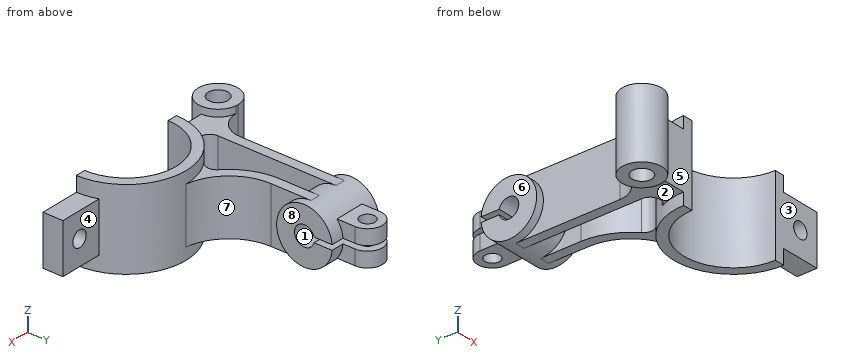
```python
from build123d import *

# Parameters (mm, degrees)
BOSS_EXTRUDE1_DEPTH = 40
SKETCH1_3_R         = 9.999999999999993
BOSS_EXTRUDE2_DEPTH = 35
BOSS_EXTRUDE3_DEPTH = 28
BOSS_EXTRUDE4_DEPTH = 25
SKETCH3_R           = 8.000000000000012
CUT_EXTRUDE1_DEPTH  = 67
SKETCH8_R           = 27.999999999999996
BOSS_EXTRUDE5_DEPTH = 28
SKETCH9_R           = 7.500000000000014
BOSS_EXTRUDE6_DEPTH = 17.5
SKETCH10_R          = 10.000000000000004
CUT_EXTRUDE3_DEPTH  = 60
SKETCH10_4_R        = 10.000000000000004
CUT_EXTRUDE4_DEPTH  = 60


with BuildPart() as part:
    # Sketch1 → Boss-Extrude1 (new, symmetric)
    with BuildSketch(Plane.XY):
        with BuildLine():
            ThreePointArc((50, 0), (3.06e-15, 50), (-50, 0))
            Line((-50, 0), (-60, 0))
            ThreePointArc((-60, 0), (3.67e-15, 60), (60, 0))
            Line((60, 0), (50, 0))
        make_face()
    extrude(amount=BOSS_EXTRUDE1_DEPTH, both=True)



with BuildPart() as body_2:
    # Sketch1<3> → Boss-Extrude2 (new, symmetric)
    with BuildSketch(Plane.XY):
        with BuildLine():
            ThreePointArc((-110, 19.999999999999986), (-124.14213562373095, -14.142135623730939), (-90.00000000000001, -4.9e-15))
            ThreePointArc((-90.00000000000001, 0), (-95.13196534092553, 13.376903430037897), (-107.894154537656, 19.88882638288958))
            ThreePointArc((-107.894154537656, 19.888826382889572), (-108.94824999295787, 19.92219950575522), (-110, 20))
        make_face()
        with Locations((-110, 0)):
            Circle(SKETCH1_3_R, mode=Mode.SUBTRACT)
    extrude(amount=BOSS_EXTRUDE2_DEPTH, both=True)


with BuildPart() as part_1:
    add(part.part)

    add(body_2.part)  # Boss-Extrude3 merges body 2
    # Sketch1<6> → Boss-Extrude3 (add, symmetric)
    with BuildSketch(Plane.XY):
        with BuildLine():
            ThreePointArc((-32.98168393227754, 65.04935068656462), (-29.729511757993123, 56.976796834196755), (-34.03450339822838, 49.413081045771484))
            ThreePointArc((-34.034503398228374, 49.413081045771484), (-17.821547874044366, 57.29216727767544), (-1.66e-15, 59.99999999999999))
            ThreePointArc((-1.78e-15, 59.99999999999999), (-30.50166992482464, 76.80795981518852), (-42.63026373834409, 109.45388748555197))
            Line((-42.630263738344084, 109.45388748555196), (-42.63026373834409, 150))
            Line((-42.63026373834409, 150), (-52.63026373834409, 150))
            Line((-52.63026373834409, 150), (-52.63026373834409, 139.99999999999997))
            Line((-52.63026373834409, 139.99999999999997), (-52.630263738344084, 109.45388748555197))
            ThreePointArc((-52.63026373834408, 109.45388748555197), (-47.498675468756, 85.17514381579021), (-32.981683932277534, 65.04935068656462))
        make_face()
        with BuildLine():
            Line((-90, -3.21e-15), (-60, 0))
            ThreePointArc((-60, -3.31e-15), (-58.39942205303789, 13.766172448111766), (-53.68308320429493, 26.797883828406057))
            ThreePointArc((-53.683083204294945, 26.79788382840606), (-64.92462581302938, 21.530960790967427), (-72.63026373834407, 31.26419779980706))
            Line((-72.63026373834407, 31.264197799807064), (-72.6302637383441, 139.99999999999997))
            Line((-72.6302637383441, 139.99999999999997), (-72.6302637383441, 150))
            Line((-72.6302637383441, 150), (-82.63026373834408, 150))
            Line((-82.63026373834408, 150), (-82.63026373834408, 44.88743357701219))
            ThreePointArc((-82.63026373834407, 44.88743357701218), (-90.04614121236624, 27.116709478332382), (-107.894154537656, 19.888826382889572))
            ThreePointArc((-107.894154537656, 19.88882638288958), (-95.13196534092553, 13.376903430037897), (-90.00000000000001, 0))
        make_face()
    extrude(amount=BOSS_EXTRUDE3_DEPTH, both=True)

    # Sketch1<7> → Boss-Extrude4 (add, symmetric)
    with BuildSketch(Plane.XY):
        with BuildLine():
            ThreePointArc((56.568542494923804, 19.999999999999993), (59.13591357920932, 10.146118723545761), (60, 0))
            Line((60, 0), (100, 0))
            Line((100, 0), (100, 20))
            Line((100, 20), (56.568542494923804, 19.999999999999993))
        make_face()
    extrude(amount=BOSS_EXTRUDE4_DEPTH, both=True)

    # Sketch3 → Cut-Extrude1 (cut)
    with BuildSketch(Plane(origin=(-3.2e-15, 19.999999999999982, 0), x_dir=(1, 1.6e-16, 0), z_dir=(-1.6e-16, 1, 0))):
        with Locations(Location((80, 0, 0), (0, 0, 180))):
            Circle(SKETCH3_R)
    extrude(amount=-CUT_EXTRUDE1_DEPTH, mode=Mode.SUBTRACT)

    # Sketch8 → Boss-Extrude5 (add, symmetric)
    with BuildSketch(Plane(origin=(-62.630263738344055, -1.072e-14, 0), x_dir=(0, 0, -1), z_dir=(1, 1.7e-16, 0))):
        with Locations(Location((0, 150, 0), (0, 0, 90))):
            Circle(SKETCH8_R)
    extrude(amount=BOSS_EXTRUDE5_DEPTH, both=True)

    # Sketch9 → Boss-Extrude6 (add, symmetric)
    with BuildSketch(Plane.XY):
        with BuildLine():
            Line((-77.63026373834407, 190), (-77.63026373834407, 170))
            Line((-77.63026373834407, 170), (-47.63026373834407, 170))
            Line((-47.63026373834407, 170), (-47.63026373834407, 190))
            ThreePointArc((-47.63026373834407, 190), (-62.63026373834407, 205), (-77.63026373834407, 190))
        make_face()
        with Locations((-62.63026373834407, 190)):
            Circle(SKETCH9_R, mode=Mode.SUBTRACT)
    extrude(amount=BOSS_EXTRUDE6_DEPTH, both=True)

    # Sketch10 → Cut-Extrude3 (cut)
    with BuildSketch(Plane(origin=(-34.630263738344055, -5.93e-15, 0), x_dir=(0, 0, -1), z_dir=(1, 1.7e-16, 0))):
        with Locations(Location((0, 150, 0), (0, 0, 90))):
            Circle(SKETCH10_R)
    extrude(amount=-CUT_EXTRUDE3_DEPTH, mode=Mode.SUBTRACT)

    # Sketch10<4> → Cut-Extrude4 (cut)
    with BuildSketch(Plane(origin=(-34.630263738344055, -5.93e-15, 0), x_dir=(0, 0, -1), z_dir=(1, 1.7e-16, 0))):
        with Locations((0, 150)):
            Circle(SKETCH10_4_R)
        Polygon((-2.5, 150), (2.5, 150), (2.5000000000000004, 205.00000000000003), (-2.5, 205.00000000000003), align=None)
    extrude(amount=-CUT_EXTRUDE4_DEPTH, mode=Mode.SUBTRACT)


solid = part_1.part
```
Part model, mm, in its own coordinate system. Face numbers are marked on the shaded views. A direction names the side the tool comes from. Give positions to 0.01 mm unless a question says otherwise; leave off trailing zeros. Order: outer loops, then holes, each group sorted by start corner. A loop starts at its lowest first (then second) coordinate and runs counter-clockwise, first axis right, second up. Notation, with made-up numbers: M 7,18.5 L 53,18.5 A7 cw 53,24.5 Z; hole C 68.5,-13 d8. An arc over 180 degrees is marked long. Use a Markdown table: item, result. Add a question column.
(1) Saw through at C-C, the plane z = 20.5. Give the cut face in (x, y), and give its area (3 significant figures).
(2) 3-axis set-ups, long thin cutter, end or side, ignore diameter. For the marked faces 5, 6, 7 and 8: which of +Z, -Z, +X, -X, +Y, -Y reach the whole face in a straight line?
(3) Saw through at D-D, the plane x = 21.5. Give the cut face in (y, z).
(4) Drop flat-ended pins along their axis: P1, Ø9, axis at x = -61, y = 187, coming from the +Z side; P2, Ø13.5, axis at x = -61, y = 193, coming from the -Z side; P3, Ø12, axis at y = 182.5, z = 10.5, coming from the -X side. Give the stop position or say it passes through.
(5) Mould opens along Y. For the marked faces 1, 2, 3 and 4 say: +Y half, -Y half, draft (parallel to the pull), parting line (faces both ways), or undercut.
(6) Probe line 1 along Y through (x, z) = (-110, -31.5); line 2 along Z through (x, y) = (80, 9.25); line 3 along Z through (x, y) = (-61, 150). List the from-to ranges inside material, lowest first. Write a range as [from, to].
(7) Saw through at B-B, the plane y = 41.5. Give the cut face in (x, z).
(8) Saw through at A-A, the plane x = 80. Give the cut face in (y, z), and give its area (3 significant figures).
Answer key:
| question | item | result |
|---|---|---|
| 1 | outline | M -110,20 A20 ccw long -90,0 L -50,0 A50 cw 50,0 L 100,0 L 100,20 L 56.57,20 A60 ccw 0,60 A50 cw -42.63,109.45 L -42.63,130.93 L -34.63,130.93 L -34.63,169.07 L -90.63,169.07 L -90.63,130.93 L -82.63,130.93 L -82.63,44.89 A25 cw Z; hole C -110,0 d20; hole M -72.63,31.26 A10 ccw -53.68,26.8 A60 cw -34.03,49.41 A10 ccw -32.98,65.05 A60 cw -52.63,109.45 L -52.63,130.93 L -72.63,130.93 Z |
| 1 | area | 8,550 mm^2 |
| 2 | face 5 | +Z, -Z, +X, -Y |
| 2 | face 6 | +Z, -Z, -X, +Y |
| 2 | face 7 | +Z, -Z, +X |
| 2 | face 8 | +Z, -Z, +X, +Y |
| 3 | outline | M 45.14,-40 L 56.02,-40 L 56.02,40 L 45.14,40 Z |
| 4 | P1 | z = 17.5 |
| 4 | P2 | z = -17.5 |
| 4 | P3 | x = -77.63 |
| 5 | face 1 | undercut |
| 5 | face 2 | draft |
| 5 | face 3 | -Y half |
| 5 | face 4 | +Y half |
| 6 | line 1 | [-20, -10], [10, 20] |
| 6 | line 2 | [-25, -8], [8, 25] |
| 6 | line 3 | [-28, -10], [10, 28] |
| 7 | outline | M -82.86,-28 L -72.63,-28 L -72.63,28 L -82.86,28 Z; M -43.33,-40 L -27.89,-40 L -27.89,40 L -43.33,40 Z; M 27.89,-40 L 43.33,-40 L 43.33,40 L 27.89,40 Z |
| 8 | outline | M 0,-25 L 20,-25 L 20,-8 L 0,-8 Z; M 0,8 L 20,8 L 20,25 L 0,25 Z |
| 8 | area | 680 mm^2 |
